from build123d import *

# Parameters (mm, degrees)
EXTRUDE_2_DEPTH      = 160
SKETCH_20_W          = 20
SKETCH_20_H          = 4
EXTRUDE_5_DEPTH      = 105
SKETCH_24_R          = 1.5
EXTRUDE_7_DEPTH      = 2.5
SKETCH_25_W          = 203
SKETCH_25_H          = 2.5
CUT_EXTRUDE_16_DEPTH = 280.937939551
SKETCH_27_W          = 37.304830233
SKETCH_27_H          = 160
EXTRUDE_8_DEPTH      = 5
CUT_EXTRUDE_17_REACH = 214.095
SKETCH_28_R          = 1.6
SKETCH_28_R_2        = 2.5
SKETCH_29_W          = 20
SKETCH_29_H          = 3
EXTRUDE_9_DEPTH      = 20
SKETCH_30_R          = 9
CUT_EXTRUDE_18_DEPTH = 3
SKETCH_31_W          = 30
SKETCH_31_H          = 10
CUT_EXTRUDE_19_DEPTH = 5.6
FILLET_1_R           = 2
FILLET_2_R           = 2
FILLET_3_R           = 2
CUT_EXTRUDE_20_DEPTH = 10
FILLET_4_R           = 1.7


with BuildPart() as part:
    # Sketch 1 → Extrude 2 (new body)
    with BuildSketch(Plane.XY):
        Polygon((0, 0), (203, 0), (203, 2.5), (126.5, 2.5), (124, 2.5), (81.5, 2.5), (79, 2.5), (0, 2.5), align=None)
    extrude(amount=EXTRUDE_2_DEPTH)

    # Sketch 20 → Extrude 5 (add)
    with BuildSketch(Plane(origin=(0, 2.5, 0), x_dir=(1, 0, 0), z_dir=(0, 1, 0))):
        with Locations((67.115040288, -158)):
            Rectangle(SKETCH_20_W, SKETCH_20_H)
        with Locations((67.115040288, -2)):
            Rectangle(SKETCH_20_W, SKETCH_20_H)
    extrude(amount=EXTRUDE_5_DEPTH)

    # Sketch 24 → Extrude 7 (add)
    # profile 1 of 2: a face of its own
    with BuildSketch(Plane(origin=(0, 2.5, 0), x_dir=(1, 0, 0), z_dir=(0, 1, 0))):
        Polygon((57.115040288, -4), (77.115040288, -4), (77.115040288, -24), (63.211726749, -24), (63.211726749, -18.265887292), (57.115040288, -18.265887292), align=None)
        with Locations(Location((72.115040288, -9, 0), (0, 0, 270))):
            Circle(SKETCH_24_R, mode=Mode.SUBTRACT)
        with Locations(Location((67.115040288, -14, 0), (0, 0, 270))):
            Circle(SKETCH_24_R, mode=Mode.SUBTRACT)
        with Locations(Location((62.115040288, -9, 0), (0, 0, 90))):
            Circle(SKETCH_24_R, mode=Mode.SUBTRACT)
        with Locations(Location((72.115040288, -19, 0), (0, 0, 90))):
            Circle(SKETCH_24_R, mode=Mode.SUBTRACT)
    # profile 2 of 2: a face of its own
    with BuildSketch(Plane(origin=(0, 2.5, 0), x_dir=(1, 0, 0), z_dir=(0, 1, 0))):
        Polygon((63.211726749, -136), (77.115040288, -136), (77.115040288, -156), (57.115040288, -156), (57.115040288, -141.734112708), (63.211726749, -141.734112708), align=None)
        with Locations(Location((67.115040288, -146, 0), (0, 0, 90))):
            Circle(SKETCH_24_R, mode=Mode.SUBTRACT)
        with Locations(Location((72.115040288, -141, 0), (0, 0, 270))):
            Circle(SKETCH_24_R, mode=Mode.SUBTRACT)
        with Locations(Location((72.115040288, -151, 0), (0, 0, 90))):
            Circle(SKETCH_24_R, mode=Mode.SUBTRACT)
        with Locations(Location((62.115040288, -151, 0), (0, 0, 270))):
            Circle(SKETCH_24_R, mode=Mode.SUBTRACT)
    extrude(amount=EXTRUDE_7_DEPTH)

    # Sketch 25 → Cut-Extrude 16 (cut, through all)
    with BuildSketch(Plane.XY.offset(160)):
        with Locations((101.5, 1.25)):
            Rectangle(SKETCH_25_W, SKETCH_25_H)
    extrude(amount=-CUT_EXTRUDE_16_DEPTH, mode=Mode.SUBTRACT)


with BuildPart() as cut_extrude_16_piece_1:
    # of the separate pieces the step leaves, piece 1, a body of its own (cut_extrude_16_pieces)
    add(part.part.solids().sort_by_distance((57.115040288, 2.5, 0))[0])



with BuildPart() as cut_extrude_16_piece_2:
    # of the separate pieces the step leaves, piece 2, a body of its own (cut_extrude_16_pieces)
    add(part.part.solids().sort_by_distance((57.115040288, 2.5, 160))[0])


with BuildPart() as cut_extrude_16_piece_1_1:
    add(cut_extrude_16_piece_1.part)

    add(cut_extrude_16_piece_2.part)  # Extrude 8 merges Cut-Extrude 16 piece 2
    # Sketch 27 → Extrude 8 (add)
    with BuildSketch(Plane(origin=(0, 107.5, 0), x_dir=(1, 0, 0), z_dir=(0, 1, 0))):
        with Locations((66.694824847, -80)):
            Rectangle(SKETCH_27_W, SKETCH_27_H)
    extrude(amount=EXTRUDE_8_DEPTH)

    # Sketch 28 → Cut-Extrude 17 (cut, up to next)
    with BuildSketch(Plane(origin=(0, 112.5, 0), x_dir=(1, 0, 0), z_dir=(0, 1, 0)), mode=Mode.PRIVATE) as cut_extrude_17_sk1:
        with Locations(Location((61.867974578, -75, 0), (0, 0, 270))):
            Circle(SKETCH_28_R)
    cut_extrude_17_tool1 = extrude(cut_extrude_17_sk1.sketch, amount=-CUT_EXTRUDE_17_REACH, mode=Mode.PRIVATE) & cut_extrude_16_piece_1_1.part
    # Sketch 28 → Cut-Extrude 17 (cut, up to next)
    with BuildSketch(Plane(origin=(0, 112.5, 0), x_dir=(1, 0, 0), z_dir=(0, 1, 0)), mode=Mode.PRIVATE) as cut_extrude_17_sk2:
        with Locations(Location((61.867974578, -85, 0), (0, 0, 270))):
            Circle(SKETCH_28_R)
    cut_extrude_17_tool2 = extrude(cut_extrude_17_sk2.sketch, amount=-CUT_EXTRUDE_17_REACH, mode=Mode.PRIVATE) & cut_extrude_16_piece_1_1.part
    # Sketch 28 → Cut-Extrude 17 (cut, up to next)
    with BuildSketch(Plane(origin=(0, 112.5, 0), x_dir=(1, 0, 0), z_dir=(0, 1, 0)), mode=Mode.PRIVATE) as cut_extrude_17_sk3:
        with Locations(Location((66.694824846, -80, 0), (0, 0, 270))):
            Circle(SKETCH_28_R_2)
    cut_extrude_17_tool3 = extrude(cut_extrude_17_sk3.sketch, amount=-CUT_EXTRUDE_17_REACH, mode=Mode.PRIVATE) & cut_extrude_16_piece_1_1.part
    # Sketch 28 → Cut-Extrude 17 (cut, up to next)
    with BuildSketch(Plane(origin=(0, 112.5, 0), x_dir=(1, 0, 0), z_dir=(0, 1, 0)), mode=Mode.PRIVATE) as cut_extrude_17_sk4:
        with Locations(Location((71.521675114, -75, 0), (0, 0, 270))):
            Circle(SKETCH_28_R)
    cut_extrude_17_tool4 = extrude(cut_extrude_17_sk4.sketch, amount=-CUT_EXTRUDE_17_REACH, mode=Mode.PRIVATE) & cut_extrude_16_piece_1_1.part
    # Sketch 28 → Cut-Extrude 17 (cut, up to next)
    with BuildSketch(Plane(origin=(0, 112.5, 0), x_dir=(1, 0, 0), z_dir=(0, 1, 0)), mode=Mode.PRIVATE) as cut_extrude_17_sk5:
        with Locations(Location((71.521675114, -85, 0), (0, 0, 270))):
            Circle(SKETCH_28_R)
    cut_extrude_17_tool5 = extrude(cut_extrude_17_sk5.sketch, amount=-CUT_EXTRUDE_17_REACH, mode=Mode.PRIVATE) & cut_extrude_16_piece_1_1.part
    # Sketch 28 → Cut-Extrude 17 (cut, up to next)
    with BuildSketch(Plane(origin=(0, 112.5, 0), x_dir=(1, 0, 0), z_dir=(0, 1, 0)), mode=Mode.PRIVATE) as cut_extrude_17_sk6:
        with BuildLine():
            Line((77.92150076, -141.671137219), (77.92150076, -116.497525995))
            ThreePointArc((77.92150076, -116.497525995), (66.694824846, -105.270850081), (55.468148932, -116.497525995))
            Line((55.468148932, -116.497525995), (55.468148932, -141.671137219))
            ThreePointArc((55.468148932, -141.671137219), (66.694824846, -152.897813133), (77.92150076, -141.671137219))
        make_face()
    cut_extrude_17_tool6 = extrude(cut_extrude_17_sk6.sketch, amount=-CUT_EXTRUDE_17_REACH, mode=Mode.PRIVATE) & cut_extrude_16_piece_1_1.part
    add(cut_extrude_17_tool1.solids().sort_by_distance((61.867975, 112.5, 75))[0], mode=Mode.SUBTRACT)
    add(cut_extrude_17_tool2.solids().sort_by_distance((61.867975, 112.5, 85))[0], mode=Mode.SUBTRACT)
    add(cut_extrude_17_tool3.solids().sort_by_distance((66.694825, 112.5, 80))[0], mode=Mode.SUBTRACT)
    add(cut_extrude_17_tool4.solids().sort_by_distance((71.521675, 112.5, 75))[0], mode=Mode.SUBTRACT)
    add(cut_extrude_17_tool5.solids().sort_by_distance((71.521675, 112.5, 85))[0], mode=Mode.SUBTRACT)
    add(cut_extrude_17_tool6.solids().sort_by_distance((66.694825, 112.5, 129.084332))[0], mode=Mode.SUBTRACT)

    # Sketch 29 → Extrude 9 (add)
    with BuildSketch(Plane(origin=(0, 112.5, 0), x_dir=(1, 0, 0), z_dir=(0, 1, 0))):
        with Locations((66.694824846, -21.5)):
            Rectangle(SKETCH_29_W, SKETCH_29_H)
    extrude(amount=EXTRUDE_9_DEPTH)

    # Sketch 30 → Cut-Extrude 18 (cut)
    with BuildSketch(Plane(origin=(0, 0, 20), x_dir=(-1, 0, 0), z_dir=(0, 0, -1))):
        with Locations((-66.694824846, 122.5)):
            Circle(SKETCH_30_R)
    extrude(amount=-CUT_EXTRUDE_18_DEPTH, mode=Mode.SUBTRACT)

    # Sketch 31 → Cut-Extrude 19 (cut)
    with BuildSketch(Plane(origin=(0, 112.5, 0), x_dir=(1, 0, 0), z_dir=(0, 1, 0))):
        with Locations((66.694824846, -15)):
            Rectangle(SKETCH_31_W, SKETCH_31_H)
        with Locations((66.694824846, -28)):
            Rectangle(SKETCH_31_W, SKETCH_31_H)
    extrude(amount=-CUT_EXTRUDE_19_DEPTH, mode=Mode.SUBTRACT)

    # Fillet 1
    fillet_1_edges = [cut_extrude_16_piece_1_1.edges().sort_by_distance(p)[0] for p in [
        (85.347239963, 107.5, 80),
        (48.04240973, 107.5, 80),
        (85.347239963, 112.5, 80),
        (66.694824846, 112.5, 0),
        (48.04240973, 112.5, 80),
        (66.694824846, 112.5, 160),
    ]]
    fillet(fillet_1_edges, radius=FILLET_1_R)

    # Fillet 2
    fillet_2_edges = [cut_extrude_16_piece_1_1.edges().sort_by_distance(p)[0] for p in [
        (57.115040288, 55, 160),
        (57.115040288, 56.25, 156),
        (77.115040288, 56.25, 156),
        (77.115040288, 55, 160),
        (77.115040288, 56.25, 4),
        (77.115040288, 55, 0),
        (57.115040288, 56.25, 4),
        (57.115040288, 55, 0),
    ]]
    fillet(fillet_2_edges, radius=FILLET_2_R - 0.0001)  # a hair under: the kernel refuses the full size

    # Fillet 3
    fillet_3_edges = [cut_extrude_16_piece_1_1.edges().sort_by_distance(p)[0] for p in [
        (66.694824846, 112.5, 152.897813133),
        (77.92150076, 112.5, 129.084331607),
        (66.694824846, 112.5, 105.270850081),
        (55.468148932, 112.5, 129.084331607),
        (77.92150076, 107.5, 129.084331607),
        (66.694824846, 107.5, 152.897813133),
        (55.468148932, 107.5, 129.084331607),
        (66.694824846, 107.5, 105.270850081),
    ]]
    fillet(fillet_3_edges, radius=FILLET_3_R)

    # Sketch 33 → Cut-Extrude 20 (cut)
    with BuildSketch(Plane(origin=(0, 112.5, 0), x_dir=(1, 0, 0), z_dir=(0, 1, 0))):
        with BuildLine():
            Line((53.468148932, -43.502474005), (53.468148932, -33))
            Line((53.468148932, -33), (79.92150076, -33))
            Line((79.92150076, -33), (79.92150076, -43.502474005))
            ThreePointArc((79.92150076, -43.502474005), (66.694824846, -56.729149919), (53.468148932, -43.502474005))
        make_face()
    extrude(amount=-CUT_EXTRUDE_20_DEPTH, mode=Mode.SUBTRACT)

    # Fillet 4
    fillet_4_edges = [cut_extrude_16_piece_1_1.edges().sort_by_distance(p)[0] for p in [
        (66.694824846, 107.5, 56.729149919),
        (79.92150076, 107.5, 38.251237003),
        (53.468148932, 107.5, 38.251237003),
        (53.468148932, 112.5, 38.251237003),
        (66.694824846, 112.5, 56.729149919),
        (79.92150076, 112.5, 38.251237003),
    ]]
    fillet(fillet_4_edges, radius=FILLET_4_R)


solid = cut_extrude_16_piece_1_1.part
For this review, take the finished solid that the model builds, in its own axes (mm). A direction names the side the tool comes from. Give positions to 0.01 mm unless a question says otherwise; leave off trailing zeros. Loops run counter-clockwise (first coordinate to the right, second up) from the corner with the lowest first, then second, coordinate; pieces in that order, holes last. Notation, with made-up numbers: M -36,-3 L 17,-3 A22 ccw 17,25 Z; hole C -38.5,65 d2. An arc over 180 degrees is marked long. Answer as a JSON object with one key per item and string values. Group by question number.
Q1. Insertion check: P1, Ø12, axis at x = 64, z = 94, coming from the -Y side; P2, Ø2, axis at y = 3, z = 140, coming from the -X side; P3, Ø22, axis at x = 64.5, z = 152, coming from the +Y side; P4, Ø24, axis at y = 46.5, z = 143.5, coming from the +X side. Each pin has a flat end and moves straight along its axis. Give the tip position at first contact, or say it passes through.
Q2. Add section A-A on z = 80. Give the boundary of the cut face in (x, y), and give its area (3 significant figures).
Q3. Add section C-C on z = 27. Give the boundary of the cut face in (x, y), and give its area (3 significant figures).
Q4. For probe 1 along X at (y, z) = (110.45, 75); probe 2 along X at (y, z) = (3, 9); probe 3 along Z at (x, y) = (67.5, 72), list the stretches that pass through material, from the lowest coordinate up. Write a range as [from, to].
Q5. Add section D-D on y = 119. Give the boundary of the cut face in (x, z), and give its area (3 significant figures).
Q6. Tool access review of faces 1 (the flat face through (51.695, 110, 28)), 2 (the flat face through (70, 112, 23)), 3 (the flat face through (67, 56, 156)): name each direction out of +Z, -Z, +X, -X, +Y, -Y from which nothing blocks a thin tool from reaching the whole face with its end or side.
Q7. Mouldability with a two-part tool opening along Y and no side actions: class faces 4 (the flat face through (69, 5, 13)), 5 (the cylindrical face through (73.33, 128.58, 21.48)), 6 (the flat face through (67, 2.5, 12)), 7 (the cylindrical face through (66.942, 110.007, 105.274)) as +Y half, -Y half, draft (parallel to the pull), parting line (faces both ways), or undercut.
Checked values:
{
 "1": {"P1": "y = 107.5", "P2": "x = 63.21", "P3": "y = 112.5", "P4": "through"},
 "2": {"outline": "M 48.04,109.5 A2 ccw 50.04,107.5 L 64.19,107.5 L 64.19,112.5 L 50.04,112.5 A2 ccw 48.04,110.5 Z; M 69.19,107.5 L 83.35,107.5 A2 ccw 85.35,109.5 L 85.35,110.5 A2 ccw 83.35,112.5 L 69.19,112.5 Z", "area": "158 mm²"},
 "3": {"outline": "M 48.04,109.5 A2 ccw 50.04,107.5 L 51.69,107.5 L 51.69,112.5 L 50.04,112.5 A2 ccw 48.04,110.5 Z; M 81.69,107.5 L 83.35,107.5 A2 ccw 85.35,109.5 L 85.35,110.5 A2 ccw 83.35,112.5 L 81.69,112.5 Z", "area": "33.1 mm²"},
 "4": {"probe 1": "[48.04, 60.27], [63.47, 69.92], [73.12, 85.35]", "probe 2": "[57.12, 60.62], [63.62, 70.62], [73.62, 77.12]", "probe 3": "[0, 4], [156, 160]"},
 "5": {"outline": "M 56.69,20 L 58.4,20 L 58.4,23 L 56.69,23 Z; M 74.99,20 L 76.69,20 L 76.69,23 L 74.99,23 Z", "area": "10.3 mm²"},
 "6": {"face 1": "+Y, -Y", "face 2": "+Y", "face 3": "+X, -X"},
 "7": {"face 4": "undercut", "face 5": "undercut", "face 6": "-Y half", "face 7": "draft"}
}
